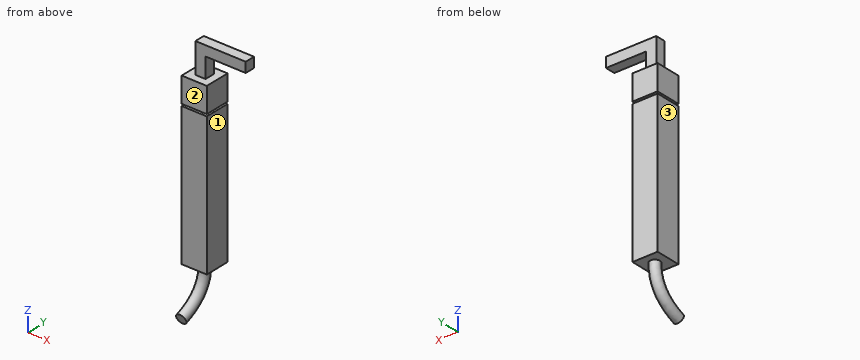
Autodesk Inventor part; units mm, degrees
ref_plane "Work Plane1" through (-4.5, 2.2217, -19.7) normal (1, 0, 0) x (0, -1, 0)
ref_plane "YZ Plane" through (0, 0, 0) normal (1, 0, 0) x (0, 1, 0)
ref_plane "XZ Plane" through (0, 0, 0) normal (0, 1, 0) x (-1, 0, 0)
sketch "Sketch1" plane through (0, 0, 0) normal (0, 1, 0) x (-1, 0, 0)
  line L0 (0, 0) -> (5, 0)
  line L1 (5, 0) -> (5, -13)
  line L2 (5, -13) -> (4, -13)
  line L3 (4, -13) -> (4, -1)
  line L4 (4, -1) -> (0, -1)
  line L5 (0, -1) -> (0, 0)
  line L6 (5.75, -3) -> (3.25, -3)
  line L7 (3.25, -3) -> (3.25, -5.5)
  line L8 (3.25, -5.5) -> (5.75, -5.5)
  line L9 (5.75, -5.5) -> (5.75, -3)
  line L10 (4.5, -1.8535) -> (4.5, -3.6396) construction
  line L11 (5.75, -5.7) -> (3.25, -5.7)
  line L12 (3.25, -5.7) -> (3.25, -19.7)
  line L13 (3.25, -19.7) -> (5.75, -19.7)
  line L14 (5.75, -19.7) -> (5.75, -5.7)
  dimension "d0" = 4
  dimension "d1" = 5
  dimension "d2" = 2.5
  dimension "d3" = 2.5
  dimension "d4" = 2
  dimension "d16" = 0.2
  dimension "d19" = 14
  dimension "d20" = 7.5
extrude "Extrusion1" add sketch "Sketch1" along normal blind 0.5 and the other way blind 0.5 contours L0 L1 L6 L3 L4 L5 | L1 L8 L3 L6 | L1 L11 L3 L8 | L1 L2 L3 L11
extrude "Extrusion2" add sketch "Sketch1" against normal blind 1.25 and the other way blind 1.25 contours L6 L9 L8 L1 | L1 L8 L3 L6 | L3 L8 L7 L6 | L11 L14 L13 L12 L3 L2 L1 | L1 L2 L3 L11
sketch "Sketch2" plane through (-3.25, -1.25, -19.7) normal (0, 0, -1) x (-1, 0, 0)
  line L0 (1.25, 3.4717) -> (1.25, -1.4422) construction
ref_plane "Work Plane1" through (-4.5, 2.2217, -19.7) normal (1, 0, 0) x (0, -1, 0)
sketch "Sketch3" plane through (-4.5, 2.2217, -19.7) normal (1, 0, 0) x (0, -1, 0)
  line L0 (2.2217, 0.0174) -> (2.2217, 2.5917) construction
  line L1 (2.2217, 2.5917) -> (5.0748, 3.6547) construction
  spline S0 degree 2 poles (2.2217, 0.0174) (2.2217, 2.5917) (5.0748, 3.6547) knots 1 1 1 2 2 2
  point P0 (2.2217, -19.7)
sketch "Sketch4" plane through (-3.25, -1.25, -19.7) normal (0, 0, -1) x (-1, 0, 0)
  circle A0 centre (1.2535, 1.3137) radius 0.5
  point P0 (-3.25, 1.25)
  dimension "d22" = 1
sweep "Sweep1" add profiles "Sketch4" path "Sketch3"
properties part number "Pin-connector-angled"
Work out the finished part from the listing and answer in its coordinate system (mm). Face numbers are marked on the shaded views. A direction names the side the tool comes from. Coordinates: 2 decimals unless noted, no trailing zeros. Loops run counter-clockwise (first coordinate to the right, second up) from the corner with the lowest first, then second, coordinate; pieces in that order, holes last. Notation, with made-up numbers: (23.5, 14.5) - (43.5, 14.5) arc R10 ccw to (43.5, 21.5) - close; hole circle Ø10 at (32.25, -20.5). An arc over 180 degrees is marked (long way). Use a Markdown table: item, result.
Item 1: Find section B-B, the plane x = -2.9. Determine the outline of the cut face in (y, z), and give its area (3 significant figures).
Evaluation:
| item | result |
|---|---|
| outline | (-0.5, -1) - (0.5, -1) - (0.5, 0) - (-0.5, 0) - close |
| area | 1.00 mm2 |
Item 2: Find section C-C, the plane z = -12.5. Determine the outline of the cut face in (x, y), and give its area (3 significant figures).
Evaluation:
| item | result |
|---|---|
| outline | (-5.75, -1.25) - (-3.25, -1.25) - (-3.25, 1.25) - (-5.75, 1.25) - close |
| area | 6.25 mm2 |
Item 3: For the marked faces 1, 2 and 3, determine the directions among +Z, -Z, +X, -X, +Y, -Y from which every point of the face is accessible in a straight line to the end or side of a thin tool.
Evaluation:
| item | result |
|---|---|
| face 1 | -Z, +X, +Y, -Y |
| face 2 | +Z, +X, -X, -Y |
| face 3 | +Z, -Z, -X, +Y, -Y |
Item 4: Given pin 1 Ø1.2 at (x, y) = (-5, -0.5) entering from -Z; pin 2 Ø0.8 at (y, z) = (0, -2) entering from +X; pin 3 Ø1.1 at (y, z) = (0, -1) entering from -X, each flat-ended and moving along its own axis, determine where each tip first touches the part or whether it passes through.
Evaluation:
| item | result |
|---|---|
| pin 1 | stops at z = -22.95 |
| pin 2 | stops at x = -4 |
| pin 3 | stops at x = -5 |
Item 5: Consider probe 1 along Z at (x, y) = (-3.55, -0.45); probe 2 along X at (y, z) = (0.7, -10); probe 3 along Y at (x, z) = (-4.95, -19). Determine where each line is inside the solid, lowest interval first. Write a range as from..to.
Evaluation:
| item | result |
|---|---|
| probe 1 | z = -19.7..-5.7, -5.5..-3, -1..0 |
| probe 2 | x = -5.75..-3.25 |
| probe 3 | y = -1.25..1.25 |
Item 6: Find section A-A, the plane y = 0.85. Determine the outline of the cut face in (x, z).
Evaluation:
| item | result |
|---|---|
| outline | (-5.75, -19.7) - (-3.25, -19.7) - (-3.25, -5.7) - (-5.75, -5.7) - close; (-5.75, -5.5) - (-3.25, -5.5) - (-3.25, -3) - (-5.75, -3) - close |
